Autodesk Inventor part; units mm, degrees
ref_plane "YZ Plane" through (0, 0, 0) normal (1, 0, 0) x (0, 1, 0)
ref_plane "XZ Plane" through (0, 0, 0) normal (0, 1, 0) x (-1, 0, 0)
ref_plane "XY Plane" through (0, 0, 0) normal (0, 0, 1) x (1, 0, 0)
sketch "Sketch1" plane through (0, 0, 0) normal (0, 0, 1) x (1, 0, 0)
  line L0 (-50, 50) -> (50, 50)
  line L1 (50, 50) -> (50, -50)
  line L2 (50, -50) -> (-50, -50)
  line L3 (-50, -50) -> (-50, 50)
  line L4 (-50, 50) -> (50, -50) construction
  line L5 (50, 50) -> (-50, -50) construction
  point P0 (0, 0)
  dimension "d0" = 100
  dimension "d1" = 100
extrude "Extrusion1" add sketch "Sketch1" along normal mid plane 100
shell "Shell1" thickness 1 removed faces 1 at (16.6667, 50, -16.6667)
properties part number "test"
Build history of the part. All positions in model axes, mm. A direction names the side the tool comes from. Coordinates: 2 decimals unless noted, no trailing zeros. Order: outer loops, then holes, each group sorted by start corner. A loop starts at its lowest first (then second) coordinate and runs counter-clockwise, first axis right, second up. Notation, with made-up numbers: M -31.75,-2.5 L -7.75,-2.5 A22 cw -7.75,6.5 Z; hole C 61,46 d9. An arc over 180 degrees is marked long. One line per question, with ' | ' between items. Start each with the question number.
Q1. Saw through at B-B (z = 32.5). List the corners of the cut face in (x, y).
Q2. Saw through at A-A (y = -25). List the corners of the cut face in (x, z), then the cut area to 3 significant figures.
Q3. 3-axis set-ups, long thin cutter, end or side, ignore diameter. For faces 1 (the face through (-49, 0, -1)), 2 (the face through (-1, 1, 50)): which of +Z, -Z, +X, -X, +Y, -Y reach the whole face in a straight line?
Q4. Flat gauge pin, fed straight in: pin 1 Ø5 at (x, z) = (7.5, 1) entering from +Y. Where does the tip first touch, or does it go through?
Q5. Probe L1, parallel to Z at x = -20, y = 6; L2, parallel to Y at x = 24.5, z = 39. List the from-to ranges inside material, lowest first. Write a range as from..to.
Q6. Saw through at C-C (x = -20). List the corners of the cut face in (y, z).
Q7. Two-plate mould, pull along X, no slides. Class faces 3 (the face through (-1, 1, -50)), 4 (the face through (-1, 1, -49)), 5 (the face through (50, 1, -1)), 6 (the face through (-50, -1, -1)): +X half, -X half, draft (parallel to the pull), parting line (faces both ways), or undercut.
Check values:
1) outline: M -50,-50 L 50,-50 L 50,50 L 49,50 L 49,-49 L -49,-49 L -49,50 L -50,50 Z
2) outline: M -50,-50 L 50,-50 L 50,50 L -50,50 Z; hole M -49,-49 L 49,-49 L 49,49 L -49,49 Z | area: 396 mm2
3) face 1: +Y | face 2: +Z, +X, -X, +Y, -Y
4) pin 1: stops at y = -49
5) L1: z = -50..-49, 49..50 | L2: y = -50..-49
6) outline: M -50,-50 L 50,-50 L 50,-49 L -49,-49 L -49,49 L 50,49 L 50,50 L -50,50 Z
7) face 3: draft | face 4: undercut | face 5: +X half | face 6: -X half
